The listing builds one solid part. Answer for the finished solid, in the listing's coordinates (mm). Face numbers are marked on the shaded views. A direction names the side the tool comes from. Round coordinates to 2 decimals unless told otherwise and drop trailing zeros. Order: outer loops, then holes, each group sorted by start corner. A loop starts at its lowest first (then second) coordinate and runs counter-clockwise, first axis right, second up. Notation, with made-up numbers: M 39,71 L 91,71 A22 cw 91,84 Z; hole C -8,51.25 d4. An arc over 180 degrees is marked long. Write item = value, one per line. Start each with the question number.
(1) A cutting plane is placed at A-A, the plane x = 191.5. Determine the outline of the cut face in (y, z), and give its area (3 significant figures).
(2) A cutting plane is placed at D-D, the plane z = 60.5. Determine the outline of the cut face in (x, y), and give its area (3 significant figures).
(3) A cutting plane is placed at B-B, the plane x = 0. Determine the outline of the cut face in (y, z).
(4) Each of these flat-tipped pins is pushed along its axis until it touches: pin 1 (9 mm diameter, centred on x = 0, y = 0, fed in from +Z); pin 2 (17.5 mm diameter, centred on x = -23.5, y = -1.5, fed in from -Z); pin 3 (6 mm diameter, centred on y = 12.5, z = -12.5, fed in from -X); pin 4 (2 mm diameter, centred on y = -3.5, z = 40, fed in from -X). Where does it stop, or does it pass through?
(5) For a pull along Z with two mould halves and no side action, classify the marked faces 3, 4, 5 and 6 as released by +Z, released by -Z, zero draft, split by the parting line, or undercut.
(6) Which of the six approach directions +Z, -Z, +X, -X, +Y, -Y give full straight-line access (tool end or side, diameter ignored) to the marked faces 1 and 2?
(7) Straight lines are drawn through the part: probe 1 along Z at (x, y) = (-57.5, -2); probe 2 along Y at (x, z) = (0, -44); probe 3 along X at (y, z) = (10, 39). For each, find the intervals that lie inside material, in ascending order. Write a range as from..to.
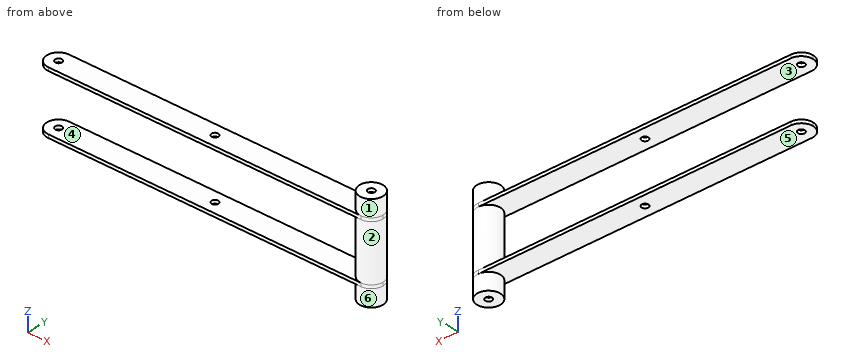
from build123d import *

# Parameters (mm, degrees)
SKETCH3_W           = 500
SKETCH3_H           = 94
BOSS_EXTRUDE3_DEPTH = 17.5
FILLET2_R           = 17.5
SKETCH4_W           = 500
SKETCH4_H           = 84
CUT_EXTRUDE2_DEPTH  = 35
SKETCH9_R           = 5
CUT_EXTRUDE4_DEPTH  = 268.660699394
SKETCH5_R           = 17.5
BOSS_EXTRUDE4_DEPTH = 72
SKETCH8_R           = 5
CUT_EXTRUDE3_DEPTH  = 5


with BuildPart() as part:
    # Sketch3 → Boss-Extrude3 (new, symmetric)
    with BuildSketch(Plane(origin=(0, 0, 0), x_dir=(1, 0, 0), z_dir=(0, 1, 0))):
        Rectangle(SKETCH3_W, SKETCH3_H)
    extrude(amount=BOSS_EXTRUDE3_DEPTH, both=True)

    # Fillet2
    fillet2_edges = [part.edges().sort_by_distance(p)[0] for p in [
        (250, -17.5, 0),
        (250, 17.5, 0),
        (-250, -17.5, 0),
        (-250, 17.5, 0),
    ]]
    fillet(fillet2_edges, radius=FILLET2_R - 0.0001)  # a hair under: the kernel refuses the full size

    # Sketch4 → Cut-Extrude2 (cut)
    with BuildSketch(Plane(origin=(0, 17.5, 0), x_dir=(1, 0, 0), z_dir=(0, 1, 0))):
        Rectangle(SKETCH4_W, SKETCH4_H)
    extrude(amount=-CUT_EXTRUDE2_DEPTH, mode=Mode.SUBTRACT)


with BuildPart() as cut_extrude2_piece_1:
    # of the separate pieces the step leaves, piece 1, a body of its own (cut_extrude2_pieces)
    add(part.part.solids().sort_by_distance((-250, -0.0001, -47))[0])


with BuildPart() as cut_extrude2_piece_2:
    # of the separate pieces the step leaves, piece 2, a body of its own (cut_extrude2_pieces)
    add(part.part.solids().sort_by_distance((-250, -0.0001, 47))[0])


with BuildPart() as cut_extrude4_tool:
    # Sketch9 → Cut-Extrude4 (new, through all)
    with BuildSketch(Plane(origin=(0, 0, -47), x_dir=(-1, 0, 0), z_dir=(0, 0, -1))):
        Circle(SKETCH9_R)
        with Locations((232.5, 0)):
            Circle(SKETCH9_R)
    extrude(amount=-CUT_EXTRUDE4_DEPTH)


with BuildPart() as cut_extrude2_piece_1_1:
    add(cut_extrude2_piece_1.part)

    # Cut-Extrude4: cut by cut_extrude4_tool
    add(cut_extrude4_tool.part, mode=Mode.SUBTRACT)



with BuildPart() as cut_extrude2_piece_2_1:
    add(cut_extrude2_piece_2.part)

    # Cut-Extrude4: cut by cut_extrude4_tool
    add(cut_extrude4_tool.part, mode=Mode.SUBTRACT)


with BuildPart() as cut_extrude2_piece_1_2:
    add(cut_extrude2_piece_1_1.part)

    add(cut_extrude2_piece_2_1.part)  # Boss-Extrude4 merges Cut-Extrude2 piece 2
    # Sketch5 → Boss-Extrude4 (add, symmetric)
    with BuildSketch(Plane.XY):
        with Locations((232.5, 0)):
            Circle(SKETCH5_R)
    extrude(amount=BOSS_EXTRUDE4_DEPTH, both=True)

    # Sketch8 → Cut-Extrude3 (cut)
    with BuildSketch(Plane(origin=(0, 0, -72), x_dir=(-1, 0, 0), z_dir=(0, 0, -1))):
        with Locations((-232.5, 0)):
            Circle(SKETCH8_R)
    cut_extrude3 = extrude(amount=-CUT_EXTRUDE3_DEPTH, mode=Mode.SUBTRACT)

    # Mirror1: Cut-Extrude3 across plane
    add(cut_extrude3.mirror(Plane.XY), mode=Mode.SUBTRACT)


solid = cut_extrude2_piece_1_2.part
Reported:
q1.outline = M -17.5,-47 L 17.5,-47 L 17.5,-42 L -17.5,-42 Z; M -17.5,42 L 17.5,42 L 17.5,47 L -17.5,47 Z
q1.area = 350 mm²
q2.outline = C 232.5,0 d35
q2.area = 962 mm²
q3.outline = M -17.5,-47 L -5,-47 L -5,-42 L -17.5,-42 Z; M -17.5,42 L -5,42 L -5,47 L -17.5,47 Z; M 5,-47 L 17.5,-47 L 17.5,-42 L 5,-42 Z; M 5,42 L 17.5,42 L 17.5,47 L 5,47 Z
q4.pin_1 = through
q4.pin_2 = -47
q4.pin_3 = 217.8
q4.pin_4 = 215.18
q5.face_3 = undercut
q5.face_4 = undercut
q5.face_5 = released by -Z
q5.face_6 = zero draft
q6.face_1 = +Z
q6.face_2 = none
q7.probe_1 = -47..-42, 42..47
q7.probe_2 = -17.5..-5, 5..17.5
q7.probe_3 = 218.14..246.86
